Source: CAD feature listing. Evaluate the final solid. Frame: model axes, mm. A direction names the side the tool comes from. Give positions to 0.01 mm unless a question says otherwise; leave off trailing zeros. Order: outer loops, then holes, each group sorted by start corner. A loop starts at its lowest first (then second) coordinate and runs counter-clockwise, first axis right, second up. Notation, with made-up numbers: M 52,-18 L 92,-18 A17 ccw 92,3 Z; hole C 27,-24 d9. An arc over 180 degrees is marked long. Return JSON: item names as keys, results as strings.
from build123d import *

# Parameters (mm, degrees)
SKETCH1_W           = 160
SKETCH1_H           = 113.333333333
BASE_EXTRUDE_DEPTH  = 100
BOSS_EXTRUDE1_DEPTH = 5
CUT_EXTRUDE1_DEPTH  = 10
CUT_EXTRUDE2_DEPTH  = 30
CUT_EXTRUDE3_DEPTH  = 20
SKETCH7_R           = 4.5
CUT_EXTRUDE4_DEPTH  = 146
CUT_EXTRUDE5_DEPTH  = 25


with BuildPart() as part:
    # Sketch1 → Base-Extrude (new body)
    with BuildSketch(Plane.XY):
        with Locations((0, 3.333333334)):
            Rectangle(SKETCH1_W, SKETCH1_H)
    extrude(amount=-BASE_EXTRUDE_DEPTH)

    # Sketch2 → Boss-Extrude1 (add)
    with BuildSketch(Plane.XY):
        with BuildLine():
            Line((-51, -20), (-9, -20))
            ThreePointArc((-9, -20), (-2.636038969, -22.636038969), (0, -29))
            Line((0, -29), (0, -31))
            ThreePointArc((0, -31), (-2.636038969, -37.363961031), (-9, -40))
            Line((-9, -40), (-51, -40))
            ThreePointArc((-51, -40), (-57.363961031, -37.363961031), (-60, -31))
            Line((-60, -31), (-60, -29))
            ThreePointArc((-60, -29), (-57.363961031, -22.636038969), (-51, -20))
        make_face()
        with BuildLine():
            Line((-51, 50), (-9, 50))
            ThreePointArc((-9, 50), (-2.636038969, 47.363961031), (0, 41))
            Line((0, 41), (0, 39))
            ThreePointArc((0, 39), (-2.636038969, 32.636038969), (-9, 30))
            Line((-9, 30), (-51, 30))
            ThreePointArc((-51, 30), (-57.363961031, 32.636038969), (-60, 39))
            Line((-60, 39), (-60, 41))
            ThreePointArc((-60, 41), (-57.363961031, 47.363961031), (-51, 50))
        make_face()
        with BuildLine():
            Line((60, -30.333333333), (40, -30.333333333))
            ThreePointArc((40, -30.333333333), (32, -38.333333333), (40, -46.333333333))
            Line((40, -46.333333333), (60, -46.333333333))
            ThreePointArc((60, -46.333333333), (68, -38.333333333), (60, -30.333333333))
        make_face()
    extrude(amount=BOSS_EXTRUDE1_DEPTH)

    # Sketch3 → Cut-Extrude1 (cut)
    with BuildSketch(Plane.XY):
        with BuildLine():
            Line((-9, 9), (-51, 9))
            ThreePointArc((-51, 9), (-60, 0), (-51, -9))
            Line((-51, -9), (-9, -9))
            ThreePointArc((-9, -9), (0, 0), (-9, 9))
        make_face()
    extrude(amount=-CUT_EXTRUDE1_DEPTH, mode=Mode.SUBTRACT)

    # Sketch4 → Cut-Extrude2 (cut)
    with BuildSketch(Plane.XY):
        with BuildLine():
            Line((20, 80), (93.333333333, 80))
            Line((93.333333333, 80), (93.333333333, 20))
            Line((93.333333333, 20), (25, 20))
            ThreePointArc((25, 20), (21.464466094, 21.464466094), (20, 25))
            Line((20, 25), (20, 80))
        make_face()
    extrude(amount=-CUT_EXTRUDE2_DEPTH, mode=Mode.SUBTRACT)

    # Sketch5 → Cut-Extrude3 (cut)
    with BuildSketch(Plane.XY.offset(-30)):
        with BuildLine():
            Line((30, 70), (98.390848549, 70))
            Line((98.390848549, 70), (98.390848549, 31))
            Line((98.390848549, 31), (35, 31))
            ThreePointArc((35, 31), (31.464466094, 32.464466094), (30, 36))
            Line((30, 36), (30, 70))
        make_face()
    extrude(amount=-CUT_EXTRUDE3_DEPTH, mode=Mode.SUBTRACT)

    # Sketch7 → Cut-Extrude4 (cut, through all)
    with BuildSketch(Plane.XY.offset(5)):
        with Locations((-50, -30)):
            Circle(SKETCH7_R)
        with Locations((-10, -30)):
            Circle(SKETCH7_R)
        with Locations((-50, 40)):
            Circle(SKETCH7_R)
        with Locations((-10, 40)):
            Circle(SKETCH7_R)
    extrude(amount=-CUT_EXTRUDE4_DEPTH, mode=Mode.SUBTRACT)

    # Sketch9 → Cut-Extrude5 (cut)
    with BuildSketch(Plane.XY):
        with BuildLine():
            Line((29, 9), (103.333333333, 9))
            Line((103.333333333, 9), (103.333333333, -20))
            Line((103.333333333, -20), (29, -20))
            ThreePointArc((29, -20), (22.636038969, -17.363961031), (20, -11))
            Line((20, -11), (20, 0))
            ThreePointArc((20, 0), (22.636038969, 6.363961031), (29, 9))
        make_face()
    extrude(amount=-CUT_EXTRUDE5_DEPTH, mode=Mode.SUBTRACT)


solid = part.part
1. Draft query along X for faces 5 (the face through (-1, 4, -100)), 6 (the face through (-30, 0, -10)), 7 (the face through (68, -38.5, 2.5)), 8 (the face through (-47.92, 36.01, -46.76)). Return one class per face: pulls with the +X half, pulls with the -X half, needs draft (parallel to the pull), parting line crosses it, or undercut.
Evaluation:
{"face 5": "needs draft", "face 6": "undercut", "face 7": "pulls with the +X half", "face 8": "undercut"}
2. Section query A-A (z = -22). Return loops of the section in (x, y).
Evaluation:
{"outline": "M -80,-53.33 L 80,-53.33 L 80,-20 L 29,-20 A9 cw 20,-11 L 20,0 A9 cw 29,9 L 80,9 L 80,20 L 25,20 A5 cw 20,25 L 20,60 L -80,60 Z; hole C -50,-30 d9; hole C -50,40 d9; hole C -10,-30 d9; hole C -10,40 d9"}
3. Ray query, probe 1 along Y at (x, z) = (-50, -78); probe 2 along Z at (x, y) = (21.5, -6.5); probe 3 along Z at (x, y) = (69.5, 26). Return the intervals inside material, ascending.
Evaluation:
{"probe 1": "y = -53.33 to -34.5, -25.5 to 35.5, 44.5 to 60", "probe 2": "z = -100 to -25", "probe 3": "z = -100 to -30"}
4. First-contact query: pin 1 (23 mm diameter, centred on x = 47.5, y = 49.5, fed in from +Z); pin 2 (5 mm diameter, centred on y = 47, z = -25, fed in from +X); pin 3 (15 mm diameter, centred on x = 40, z = -15, fed in from +Y). Flat tips, straight axial feed; report the tip coordinate or a pass-through.
Evaluation:
{"pin 1": "stops at z = -50", "pin 2": "stops at x = 20", "pin 3": "stops at y = 20"}
5. Section query B-B (y = -43). Return loops of the section in (x, z), then the cut area to 3 significant figures.
Evaluation:
{"outline": "M -80,-100 L 80,-100 L 80,0 L 66.5,0 L 66.5,5 L 33.5,5 L 33.5,0 L -80,0 Z", "area": "16,200 mm^2"}
6. Set-up query: faces 1 (the face through (50, -46.333, 2)), 2 (the face through (-2.566, 32.706, 2.465)), 3 (the face through (43, 30, -30)), 4 (the face through (-30, 30, 2)). Return all of +Z, -Z, +X, -X, +Y, -Y with unobstructed straight access to the full face (end or side cutting, diameter ignored); none if empty.
Evaluation:
{"face 1": "+Z, +X, -X, -Y", "face 2": "+Z, +X", "face 3": "+Z, +X, +Y", "face 4": "+Z, +X, -X"}
7. Section query C-C (x = 8). Return loops of the section in (y, z).
Evaluation:
{"outline": "M -53.33,-100 L 60,-100 L 60,0 L -53.33,0 Z"}
